from build123d import *

# Parameters (mm, degrees)
F2_DEPTH = 25


with BuildPart() as f2:
    # F1 (on face) → F2 (new body)
    with BuildSketch(Plane.XZ):
        Polygon((9.5947289367, 12.933765538), (0, 42.278226465), (-9.4556037773, 12.933765538), align=None)
        Polygon((9.5947289367, 12.933765538), (-9.4556037773, 12.933765538), (-15.1755097815, -4.8173545596), (0.1207542754, -15.8718874525), (15.3832069723, -4.7696806626), align=None)
        Polygon((-15.1755097815, -4.8173545596), (-9.4556037773, 12.933765538), (-39.737906307, 12.933765538), align=None)
        Polygon((39.720531553, 12.933765538), (9.5947289367, 12.933765538), (15.3832069723, -4.7696806626), align=None)
        Polygon((0.1207542754, -15.8718874525), (-15.1755097815, -4.8173545596), (-24.5111901313, -33.7896458805), align=None)
        Polygon((24.8588733375, -33.7500013411), (15.3832069723, -4.7696806626), (0.1207542754, -15.8718874525), align=None)
    extrude(amount=F2_DEPTH)


solid = f2.part
Model file for the job. Use its own axes, mm. A direction names the side the tool comes from. Round coordinates to 2 decimals unless told otherwise and drop trailing zeros. Loops run counter-clockwise (first coordinate to the right, second up) from the corner with the lowest first, then second, coordinate; pieces in that order, holes last. Notation, with made-up numbers: (89, -15) - (140, -15) arc R12 ccw to (140, 5) - close; hole circle Ø1 at (43.25, 9.5). An arc over 180 degrees is marked (long way). Write each question's results on one line, items separated by ' | '.
(1) Saw through at C-C, the plane x = -21. List the corners of the cut face in (y, z).
Answer below:
outline: (-25, -31.24) - (0, -31.24) - (0, -22.89) - (-25, -22.89) - close; (-25, -0.61) - (0, -0.61) - (0, 12.93) - (-25, 12.93) - close
(2) 3-axis set-ups, long thin cutter, end or side, ignore diameter. For faces 1 (the flat face through (-24, -12, 12.934)), 2 (the flat face through (20.2, -12.3, -19.5)), 3 (the flat face through (-27.629, -12.325, 4.182)): which of +Z, -Z, +X, -X, +Y, -Y reach the whole face in a straight line?
Answer below:
face 1: +Z, -X, +Y, -Y | face 2: +X, +Y, -Y | face 3: -X, +Y, -Y
(3) Wall check: L1, parallel to X at y = -2.75, z = -29; L2, parallel to X at y = -18.5, z = -20; L3, parallel to Z at x = -33.5, y = -21.75. Give the ranges that are in metal, low to high.
Answer below:
L1: x = -22.97 to -17.93, 18.29 to 23.31 | L2: x = -20.07 to -5.55, 5.83 to 20.36 | L3: z = 8.43 to 12.93
(4) Mould opens along X. For faces 4 (the flat face through (4.865, -12.325, 27.401)), 5 (the flat face through (-12.37, -12.32, -24.96)), 6 (the flat face through (12.32, -12.32, -24.69)), 7 (the flat face through (25, -12, 12.934)) say: released by +X, released by -X, zero draft, split by the parting line, or undercut.
Answer below:
face 4: released by +X | face 5: undercut | face 6: undercut | face 7: zero draft
(5) Saw through at A-A, the plane y = -22. List the corners of the cut face in (x, z), then the cut area to 3 significant figures.
Answer below:
outline: (-39.74, 12.93) - (-15.18, -4.82) - (-24.51, -33.79) - (0.12, -15.87) - (24.86, -33.75) - (15.38, -4.77) - (39.72, 12.93) - (9.59, 12.93) - (0, 42.28) - (-9.46, 12.93) - close | area: 1,970 mm^2
(6) Saw through at D-D, the plane z = 33.5. List the corners of the cut face in (x, y), then the cut area to 3 significant figures.
Answer below:
outline: (-2.83, -25) - (2.87, -25) - (2.87, 0) - (-2.83, 0) - close | area: 142 mm^2
(7) Pin check, flat tips, straight feed: pin 1 (10 mm diameter, centred on y = -7.5, z = 3, fed in from +X); pin 2 (7.5 mm diameter, centred on x = -26.5, y = -11, fed in from +Z); pin 3 (3 mm diameter, centred on y = -20, z = -24.5, fed in from +X). Stop position of each tip, or through.
Answer below:
pin 1: stops at x = 32.94 | pin 2: stops at z = 12.93 | pin 3: stops at x = 22.32
(8) Saw through at B-B, the plane z = -22.5. List the corners of the cut face in (x, y), then the cut area to 3 significant figures.
Answer below:
outline: (-20.87, -25) - (-8.99, -25) - (-8.99, 0) - (-20.87, 0) - close; (9.29, -25) - (21.18, -25) - (21.18, 0) - (9.29, 0) - close | area: 594 mm^2
